For this review, take the finished solid that the model builds, in its own axes (mm). Face numbers are marked on the shaded views. A direction names the side the tool comes from. Coordinates: 2 decimals unless noted, no trailing zeros. Write each loop counter-clockwise with the first axis right and the second up, starting at its lowest first coordinate (ties: lowest second). Pieces come first, ordered by that corner, then holes.
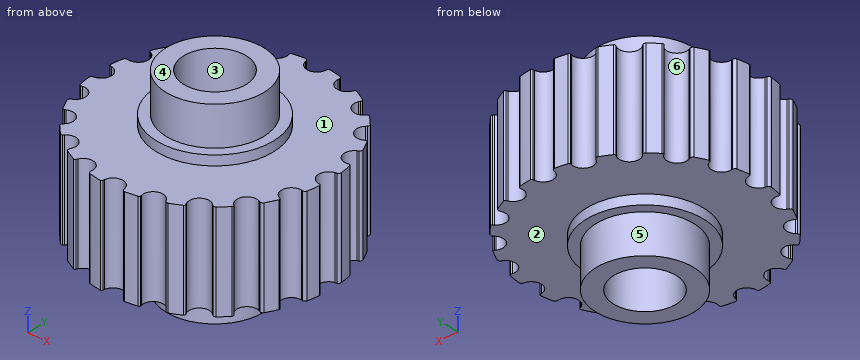
```python
from build123d import *

# Parameters (mm, degrees)
SKETCH_1_R               = 6
SKETCH_1_R_2             = 2.5
EXTRUDE_1_DEPTH          = 5
CUT_EXTRUDE_START        = -5
CUT_EXTRUDE_1_DEPTH      = 5
PATTERN_CIRCULAR_1_COUNT = 20
EXTRUDE_START            = -5.5
SKETCH_3_R               = 3
SKETCH_3_R_2             = 2.5
EXTRUDE_2_DEPTH          = 6
SKETCH_4_R               = 2.5
SKETCH_4_R_2             = 1.6
EXTRUDE_3_DEPTH          = 2
SKETCH_5_R               = 2.5
SKETCH_5_R_2             = 1.6
EXTRUDE_4_DEPTH          = 8


with BuildPart() as part:
    # Sketch 1 → Extrude 1 (new body)
    with BuildSketch(Plane.XY):
        Circle(SKETCH_1_R)
        Circle(SKETCH_1_R_2, mode=Mode.SUBTRACT)
    extrude(amount=EXTRUDE_1_DEPTH)

    # Sketch 2 → Cut-Extrude 1 (cut)
    with BuildSketch(Plane.XY.offset(5).offset(CUT_EXTRUDE_START)):
        with BuildLine():
            Line((0.511862463, 5.832363511), (0.521654336, 5.909021561))
            ThreePointArc((0.521654336, 5.909021561), (0.547634704, 5.955147301), (0.598423406, 5.970082866))
            ThreePointArc((0.598423406, 5.970082866), (-0.031806753, 5.999915694), (-0.661685201, 5.963402778))
            ThreePointArc((-0.661685201, 5.963402778), (-0.571930624, 5.939984659), (-0.520777334, 5.862604859))
            Line((-0.520777334, 5.862604859), (-0.50376482, 5.785946809))
            ThreePointArc((-0.50376482, 5.785946809), (0.023558873, 5.382262679), (0.511862463, 5.832363511))
        make_face()
    cut_extrude_1 = extrude(amount=CUT_EXTRUDE_1_DEPTH, mode=Mode.SUBTRACT)

    # Pattern Circular 1: Cut-Extrude 1 ×20 about axis
    pattern_circular_1_axis = Axis((0, 0, 0), (0, 0, 1))
    for i in range(1, PATTERN_CIRCULAR_1_COUNT):
        add(cut_extrude_1.rotate(pattern_circular_1_axis, i * 360 / PATTERN_CIRCULAR_1_COUNT), mode=Mode.SUBTRACT)

    # Sketch 3 → Extrude 2 (add)
    with BuildSketch(Plane.XY.offset(5).offset(EXTRUDE_START)):
        Circle(SKETCH_3_R)
        Circle(SKETCH_3_R_2, mode=Mode.SUBTRACT)
    extrude(amount=EXTRUDE_2_DEPTH)



with BuildPart() as body_2:
    # Sketch 4 → Extrude 3 (new body)
    with BuildSketch(Plane(origin=(0, 0, -0.5), x_dir=(-1, 0, 0), z_dir=(0, 0, -1))):
        with Locations(Location((0, 0, 0), (0, 0, 180))):
            Circle(SKETCH_4_R)
        Circle(SKETCH_4_R_2, mode=Mode.SUBTRACT)
    extrude(amount=EXTRUDE_3_DEPTH)


with BuildPart() as part_1:
    add(part.part)

    add(body_2.part)  # Extrude 4 merges body 2
    # Sketch 5 → Extrude 4 (add)
    with BuildSketch(Plane.XY.offset(-0.5)):
        Circle(SKETCH_5_R)
        with Locations(Location((0, 0, 0), (0, 0, 180))):
            Circle(SKETCH_5_R_2, mode=Mode.SUBTRACT)
    extrude(amount=EXTRUDE_4_DEPTH)


solid = part_1.part
```
1) Consider section D-D (z = -2). Give the boundary of the cut face in (x, y).
2) Consider section C-C (x = 2). Give the boundary of the cut face in (y, z), then the cut area to 3 significant figures.
3) Consider section A-A (y = 0). Give the boundary of the cut face in (x, z).
4) The part is to be moulded in two halves that separate along Y. For the marked faces 4, 5 and 6, say which applies: pulls with the +Y half, pulls with the -Y half, needs draft (parallel to the pull), parting line crosses it, or undercut.
5) For L1, parallel to Y at x = 0, z = 1.5; L2, parallel to Y at x = 0, z = 5.25, list the stretches that pass through material, from the lowest coordinate up.
6) Clearance check with flat-ended pins moving along their axes: P1, Ø1.5, axis at y = 1.5, z = 4, coming from the +X side; P2, Ø2, axis at y = -4.5, z = 5, coming from the +X side; P3, Ø5, axis at y = 4, z = 1.5, coming from the +X side. State where each tip first meets the part, or that it passes through.
7) Tool access review of the marked faces 1, 2 and 3: name each direction out of +Z, -Z, +X, -X, +Y, -Y from which nothing blocks a thin tool from reaching the whole face with its end or side.
Results:
1. outline: circle Ø5 at (0, 0); hole circle Ø3.2 at (0, 0)
2. outline: (-5.12, 0) - (-2.24, 0) - (-2.24, -0.5) - (-1.5, -0.5) - (-1.5, -2.5) - (1.5, -2.5) - (1.5, -0.5) - (2.24, -0.5) - (2.24, 0) - (5.12, 0) - (5.12, 5) - (2.24, 5) - (2.24, 5.5) - (1.5, 5.5) - (1.5, 7.5) - (-1.5, 7.5) - (-1.5, 5.5) - (-2.24, 5.5) - (-2.24, 5) - (-5.12, 5) - close
2. area: 67.7 mm2
3. outline: (-5.38, 0) - (-3, 0) - (-3, -0.5) - (-2.5, -0.5) - (-2.5, -2.5) - (-1.6, -2.5) - (-1.6, 7.5) - (-2.5, 7.5) - (-2.5, 5.5) - (-3, 5.5) - (-3, 5) - (-5.38, 5) - close; (1.6, -2.5) - (2.5, -2.5) - (2.5, -0.5) - (3, -0.5) - (3, 0) - (5.38, 0) - (5.38, 5) - (3, 5) - (3, 5.5) - (2.5, 5.5) - (2.5, 7.5) - (1.6, 7.5) - close
4. face 4: needs draft
4. face 5: parting line crosses it
4. face 6: undercut
5. L1: y = -5.38 to -1.6, 1.6 to 5.38
5. L2: y = -3 to -1.6, 1.6 to 3
6. P1: stops at x = 5.95
6. P2: stops at x = 4.5
6. P3: stops at x = 5.48
7. face 1: +Z
7. face 2: -Z
7. face 3: +Z, -Z
